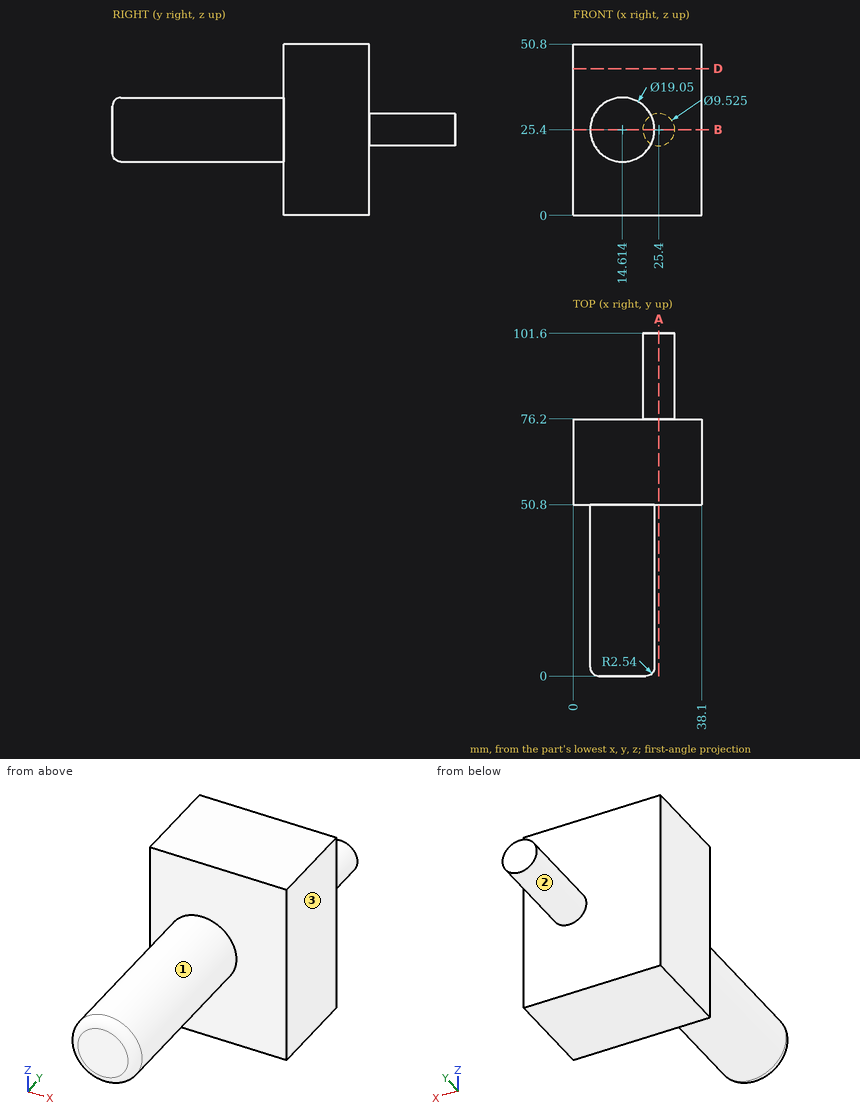
Answer from the drawing. Dimensions are ordinates in mm from the lowest x, y and z of the part. A direction names the side the tool comes from. Round coordinates to 2 decimals unless told otherwise and drop trailing zeros. Loops run counter-clockwise (first coordinate to the right, second up) from the corner with the lowest first, then second, coordinate; pieces in that order, holes last.
Q1. Section B-B on z = 25.4 is taken. Write down the section's boundary in (x, y), and give its area (3 significant figures).
Q2. Each of these flat-tipped pins is pushed along its axis until it touches: pin 1 (12 mm diameter, centred on x = 10, z = 21, fed in from +Y); pin 2 (6 mm diameter, centred on y = 88, z = 23.5, fed in from +X). Where does it stop, or does it pass through?
Q3. Consider probe 1 along Y at (x, z) = (20, 29); probe 2 along Y at (x, z) = (27, 31); probe 3 along X at (y, z) = (40.5, 32) (1 decimal). Determine where each line is inside the solid, lowest interval first.
Q4. Section A-A on x = 25.4 is taken. Write down the section's boundary in (y, z).
Q5. Which of the six approach directions +Z, -Z, +X, -X, +Y, -Y give full straight-line access (tool end or side, diameter ignored) to the marked faces 1, 2 and 3?
Q6. Section D-D on z = 43.5 is taken. Write down the section's boundary in (x, y).
Output:
1. outline: (0, 50.8) - (5.09, 50.8) - (5.09, 2.54) arc R2.54 ccw to (7.63, 0) - (21.6, 0) arc R2.54 ccw to (24.14, 2.54) - (24.14, 50.8) - (38.1, 50.8) - (38.1, 76.2) - (30.16, 76.2) - (30.16, 101.6) - (20.64, 101.6) - (20.64, 76.2) - (0, 76.2) - close
1. area: 2,170 mm2
2. pin 1: stops at y = 76.2
2. pin 2: stops at x = 30.16
3. probe 1: y = 0 to 76.2
3. probe 2: y = 50.8 to 76.2
3. probe 3: x = 7.7 to 21.5
4. outline: (50.8, 0) - (76.2, 0) - (76.2, 20.64) - (101.6, 20.64) - (101.6, 30.16) - (76.2, 30.16) - (76.2, 50.8) - (50.8, 50.8) - close
5. face 1: -Y
5. face 2: +Y
5. face 3: +Z, -Z, +X, +Y, -Y
6. outline: (0, 50.8) - (38.1, 50.8) - (38.1, 76.2) - (0, 76.2) - close
